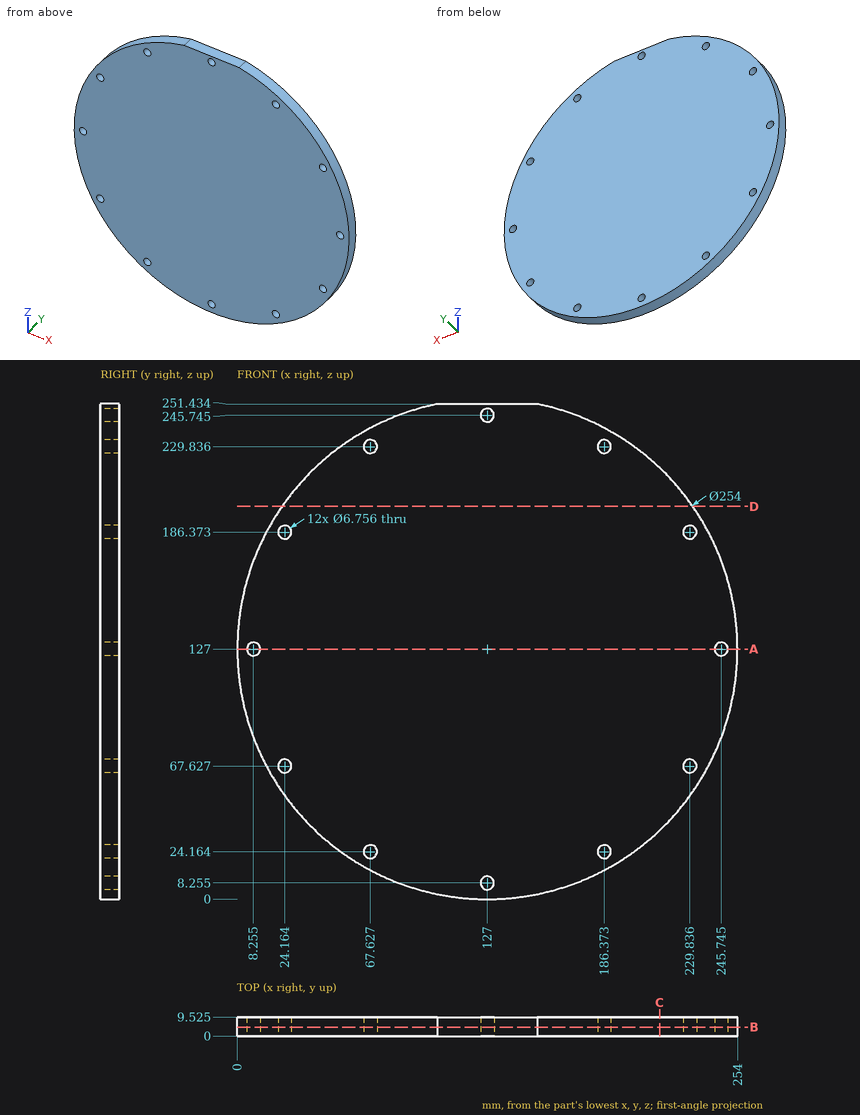
Input: dimensioned drawing with shaded views. Units: mm. Origin: part minimum x, y, z. Give positions to 0.01 mm unless a question says otherwise; leave off trailing zeros. Write each loop counter-clockwise with the first axis right and the second up, starting at its lowest first coordinate (ties: lowest second). Pieces come first, ordered by that corner, then holes. Notation, with made-up numbers: M -39.75,-4 L -17.75,-4 A31 ccw -17.75,27 Z; hole C -38,51.25 d9. An arc over 180 degrees is marked long. Write item = value, one per line. Start each with the question number.
1) Cut plane B-B on y = 4.5. Count the separate pieces of the cut face and the enclosed holes in it, then the cut area to 3 significant figures.
2) Cut plane A-A on z = 127. Return the cut outline in (x, y) (1 decimal), then the cut area to 3 significant figures.
3) Cut plane C-C on x = 214.5. Return the cut outline in (y, z) (1 decimal), then the cut area to 3 significant figures.
4) Material intervals for line 1 along X through (y, z) = (2.75, 68.5) (1 decimal); line 2 along Z through (x, y) = (232, 8.5) (1 decimal); line 3 along X through (y, z) = (6, 23.5) (1 decimal), sorted ascending. Write a range as [from, to].
5) First-contact query: pin 1 Ø3 at (x, y) = (211, 5) entering from +Z (1 decimal); pin 2 Ø1 at (y, z) = (2, 94.5) entering from -X; pin 3 Ø1.5 at (x, y) = (193, 5) entering from +Z (1 decimal). Flat tips, straight axial feed; report the tip coordinate or a pass-through.
6) Cut plane D-D on z = 199.5. Return the cut outline in (x, y) (1 decimal).
Solved:
q1.separate_pieces = 1
q1.enclosed_holes = 12
q1.area = 50,200 mm2
q2.outline = M 0,0 L 4.9,0 L 4.9,9.5 L 0,9.5 Z; M 11.6,0 L 242.4,0 L 242.4,9.5 L 11.6,9.5 Z; M 249.1,0 L 254,0 L 254,9.5 L 249.1,9.5 Z
q2.area = 2,290 mm2
q3.outline = M 0,35 L 9.5,35 L 9.5,219 L 0,219 Z
q3.area = 1,750 mm2
q4.line_1 = [14.3, 20.9], [27.4, 226.6], [233.1, 239.7]
q4.line_2 = [55.6, 65], [70.2, 183.8], [189, 198.4]
q4.line_3 = [53.4, 64.3], [70.9, 183.1], [189.7, 200.6]
q5.pin_1 = 223.6
q5.pin_2 = 4.1
q5.pin_3 = 236
q6.outline = M 22.7,0 L 231.3,0 L 231.3,9.5 L 22.7,9.5 Z
